Check sheet for the modelled part. Datum: model origin and axes. Units: mm. Round coordinates to 2 decimals unless told otherwise and drop trailing zeros. Loops run counter-clockwise (first coordinate to the right, second up) from the corner with the lowest first, then second, coordinate; pieces in that order, holes last. Notation, with made-up numbers: M -28.75,47.25 L -20.75,47.25 A30 cw -20.75,82.25 Z; hole C 43,-3.5 d8. An arc over 180 degrees is marked long. Write item = value, one per line. Start each with the question number.
(1) Cross-section at C-C on z = -49. Record the boundary of the cut face in (x, y), plus the area to 3 significant figures.
(2) Cross-section at A-A on x = 0. Record the boundary of the cut face in (y, z), plus the area to 3 significant figures.
(3) Cross-section at D-D on x = -49. Record the boundary of the cut face in (y, z).
(4) Cross-section at B-B on z = 0. Record the boundary of the cut face in (x, y).
(5) Mould release check, pull along X, two halves, no side actions. Record for faces 1 (the face through (-11.923, 0.789, 53.692)), 2 (the face through (-50.464, 0.811, -0.325)), 3 (the face through (-41, 0, -12)): pulls with the +X half, pulls with the -X half, needs draft (parallel to the pull), parting line crosses it, or undercut.
(6) Scan lines: L1, parallel to X at y = 1.15, z = 0; L2, parallel to Z at x = 34.5, y = 1.2; L3, parallel to X at y = 0.5, z = -49. Record each from-to range of solid material in increasing order. Write a range as from..to.
from build123d import *

# Parameters (mm, degrees)
SKETCH_1_R          = 55
SKETCH_1_R_2        = 42.4
EXTRUDE_1_DEPTH     = 1.6
SKETCH_2_R          = 1.5
CUT_EXTRUDE_1_DEPTH = 1.6


with BuildPart() as part:
    # 草图1 → 拉伸-薄壁1 (new body)
    with BuildSketch(Plane(origin=(0, 0, 0), x_dir=(1, 0, 0), z_dir=(0, 1, 0))):
        Circle(SKETCH_1_R)
        Circle(SKETCH_1_R_2, mode=Mode.SUBTRACT)
    extrude(amount=EXTRUDE_1_DEPTH)

    # 草图2 → 切除-拉伸1 (cut)
    with BuildSketch(Plane(origin=(0, 1.6, 0), x_dir=(1, 0, 0), z_dir=(0, 1, 0))):
        with Locations(Location((-49, 0, 0), (0, 0, 270))):
            Circle(SKETCH_2_R)
        with Locations(Location((0, 49, 0), (0, 0, 270))):
            Circle(SKETCH_2_R)
        with Locations(Location((49, 0, 0), (0, 0, 270))):
            Circle(SKETCH_2_R)
        with Locations(Location((0, -49, 0), (0, 0, 270))):
            Circle(SKETCH_2_R)
    extrude(amount=-CUT_EXTRUDE_1_DEPTH, mode=Mode.SUBTRACT)


solid = part.part
Result:
q1.outline = M -24.98,0 L -1.5,0 L -1.5,1.6 L -24.98,1.6 Z; M 1.5,0 L 24.98,0 L 24.98,1.6 L 1.5,1.6 Z
q1.area = 75.1 mm^2
q2.outline = M 0,-55 L 1.6,-55 L 1.6,-50.5 L 0,-50.5 Z; M 0,-47.5 L 1.6,-47.5 L 1.6,-42.4 L 0,-42.4 Z; M 0,42.4 L 1.6,42.4 L 1.6,47.5 L 0,47.5 Z; M 0,50.5 L 1.6,50.5 L 1.6,55 L 0,55 Z
q2.area = 30.7 mm^2
q3.outline = M 0,-24.98 L 1.6,-24.98 L 1.6,-1.5 L 0,-1.5 Z; M 0,1.5 L 1.6,1.5 L 1.6,24.98 L 0,24.98 Z
q4.outline = M -55,0 L -50.5,0 L -50.5,1.6 L -55,1.6 Z; M -47.5,0 L -42.4,0 L -42.4,1.6 L -47.5,1.6 Z; M 42.4,0 L 47.5,0 L 47.5,1.6 L 42.4,1.6 Z; M 50.5,0 L 55,0 L 55,1.6 L 50.5,1.6 Z
q5.face_1 = parting line crosses it
q5.face_2 = undercut
q5.face_3 = needs draft
q6.L1 = -55..-50.5, -47.5..-42.4, 42.4..47.5, 50.5..55
q6.L2 = -42.83..-24.65, 24.65..42.83
q6.L3 = -24.98..-1.5, 1.5..24.98
